Build history of the part. All positions in model axes, mm. A direction names the side the tool comes from. Round coordinates to 2 decimals unless told otherwise and drop trailing zeros. Order: outer loops, then holes, each group sorted by start corner. A loop starts at its lowest first (then second) coordinate and runs counter-clockwise, first axis right, second up. Notation, with made-up numbers: (1, 62.5) -> (59, 62.5) arc R10 ccw to (59, 66.5) -> close; hole circle Ø2 at (1, 7). An arc over 180 degrees is marked (long way). Use a Markdown table: item, result. Add a question column.
Item 1: Pin check, flat tips, straight feed: pin 1 (5 mm diameter, centred on x = -35.5, y = -16.5, fed in from -Z); pin 2 (4.5 mm diameter, centred on y = -19.5, z = 21.5, fed in from +X); pin 3 (14 mm diameter, centred on y = -8.5, z = 2, fed in from +X); pin 4 (12 mm diameter, centred on x = -6.5, z = 8.5, fed in from -Y). Stop position of each tip, or through.
Item 2: Slice it at C-C, the plane z = -11.5. Give the cut face in (x, y).
Item 3: Slice it at D-D, the plane y = -21.5. Give the cut face in (x, z), plus the area to 3 significant figures.
Item 4: 3-axis set-ups, long thin cutter, end or side, ignore diameter. For faces 4 (the face through (59.6, -12.52, -59.68)), 5 (the face through (-18.904, -6, 0)), 6 (the face through (21, -12.7, 0)), 7 (the face through (42.93, -12.52, 37.37)), 8 (the face through (-43.47, -12.52, 37.91)): which of +Z, -Z, +X, -X, +Y, -Y reach the whole face in a straight line?
Item 5: Slice it at B-B, the plane x = 2.5. Give the cut face in (y, z), plus the area to 3 significant figures.
Item 6: Two-plate mould, pull along Z, no slides. Class faces 1 (the face through (-37.37, -12.52, 42.93)), 2 (the face through (0, 0, 23)), 3 (the face through (0, -6, -18.904)): released by +Z, released by -Z, zero draft, split by the parting line, or undercut.
Item 7: Probe L1, parallel to X at y = -11, z = -8; L2, parallel to X at y = -23, z = 33. List the from-to ranges inside material, lowest first.
Item 8: Slice it at A-A, the plane y = -10.5. Give the cut face in (x, z).
from build123d import *

# Parameters (mm, degrees)
F0_W     = 37.8080839926
F0_H     = 37.8080839926
F1_DEPTH = 12.7
F4_DEPTH = 25.4


# Not quite as in the source:
# - the program builds the solid bodies; features that only make, move or delete a surface that nothing else refers to are left out


with BuildPart() as f1:
    # F0 (on Front) → F1 (new body)
    with BuildSketch(Plane.XZ):
        Polygon((23.9840419963, 18.4223433702), (23.9840419963, 23.9840419963), (18.4223433702, 23.9840419963), (-18.4223433702, 23.9840419963), (-23.9840419963, 23.9840419963), (-23.9840419963, 18.4223433702), (-23.9840419963, -18.4223433702), (-23.9840419963, -23.9840419963), (-18.4223433702, -23.9840419963), (18.4223433702, -23.9840419963), (23.9840419963, -23.9840419963), (23.9840419963, -18.4223433702), align=None)
        Rectangle(F0_W, F0_H, mode=Mode.SUBTRACT)
    extrude(amount=F1_DEPTH)

    # F0 (on Front) → F4 (join)
    with BuildSketch(Plane.XZ):
        with BuildLine():
            Line((-23.9840419963, 23.9840419963), (-18.4223433702, 23.9840419963))
            Line((-18.4223433702, 23.9840419963), (-44.0913446559, 49.653043282))
            ThreePointArc((-44.0913446559, 49.653043282), (-46.5728804881, 46.5728804881), (-49.653043282, 44.0913446559))
            Line((-49.653043282, 44.0913446559), (-23.9840419963, 18.4223433702))
            Line((-23.9840419963, 18.4223433702), (-23.9840419963, 23.9840419963))
        make_face()
        with BuildLine():
            ThreePointArc((-49.653043282, 44.0913446559), (-46.5728804881, 46.5728804881), (-44.0913446559, 49.653043282))
            Line((-44.0913446559, 49.653043282), (-56.85978783, 62.4214864561))
            Line((-56.85978783, 62.4214864561), (-62.4214864561, 56.85978783))
            Line((-62.4214864561, 56.85978783), (-49.653043282, 44.0913446559))
        make_face()
        with BuildLine():
            ThreePointArc((-44.0913446559, -49.653043282), (-46.5728804881, -46.5728804881), (-49.653043282, -44.0913446559))
            Line((-49.653043282, -44.0913446559), (-62.4214864561, -56.85978783))
            Line((-62.4214864561, -56.85978783), (-56.85978783, -62.4214864561))
            Line((-56.85978783, -62.4214864561), (-44.0913446559, -49.653043282))
        make_face()
        with BuildLine():
            Line((-23.9840419963, -23.9840419963), (-23.9840419963, -18.4223433702))
            Line((-23.9840419963, -18.4223433702), (-49.653043282, -44.0913446559))
            ThreePointArc((-49.653043282, -44.0913446559), (-46.5728804881, -46.5728804881), (-44.0913446559, -49.653043282))
            Line((-44.0913446559, -49.653043282), (-18.4223433702, -23.9840419963))
            Line((-18.4223433702, -23.9840419963), (-23.9840419963, -23.9840419963))
        make_face()
        with BuildLine():
            Line((49.653043282, -44.0913446559), (23.9840419963, -18.4223433702))
            Line((23.9840419963, -18.4223433702), (23.9840419963, -23.9840419963))
            Line((23.9840419963, -23.9840419963), (18.4223433702, -23.9840419963))
            Line((18.4223433702, -23.9840419963), (44.0913446559, -49.653043282))
            ThreePointArc((44.0913446559, -49.653043282), (46.5728804881, -46.5728804881), (49.653043282, -44.0913446559))
        make_face()
        with BuildLine():
            Line((62.4214864561, -56.85978783), (49.653043282, -44.0913446559))
            ThreePointArc((49.653043282, -44.0913446559), (46.5728804881, -46.5728804881), (44.0913446559, -49.653043282))
            Line((44.0913446559, -49.653043282), (56.85978783, -62.4214864561))
            Line((56.85978783, -62.4214864561), (62.4214864561, -56.85978783))
        make_face()
        with BuildLine():
            Line((56.85978783, 62.4214864561), (44.0913446559, 49.653043282))
            ThreePointArc((44.0913446559, 49.653043282), (46.5728804881, 46.5728804881), (49.653043282, 44.0913446559))
            Line((49.653043282, 44.0913446559), (62.4214864561, 56.85978783))
            Line((62.4214864561, 56.85978783), (56.85978783, 62.4214864561))
        make_face()
        with BuildLine():
            Line((18.4223433702, 23.9840419963), (23.9840419963, 23.9840419963))
            Line((23.9840419963, 23.9840419963), (23.9840419963, 18.4223433702))
            Line((23.9840419963, 18.4223433702), (49.653043282, 44.0913446559))
            ThreePointArc((49.653043282, 44.0913446559), (46.5728804881, 46.5728804881), (44.0913446559, 49.653043282))
            Line((44.0913446559, 49.653043282), (18.4223433702, 23.9840419963))
        make_face()
    extrude(amount=F4_DEPTH)


solid = f1.part
Check sheet entries:
| question | item | result |
|---|---|---|
| 1 | pin 1 | z = -43.56 |
| 1 | pin 2 | x = 29.31 |
| 1 | pin 3 | x = 23.98 |
| 1 | pin 4 | through |
| 2 | outline | (-23.98, -12.7) -> (-18.9, -12.7) -> (-18.9, 0) -> (-23.98, 0) -> close; (18.9, -12.7) -> (23.98, -12.7) -> (23.98, 0) -> (18.9, 0) -> close |
| 3 | outline | (-62.42, -56.86) -> (-56.86, -62.42) -> (-18.42, -23.98) -> (-23.98, -23.98) -> (-23.98, -18.42) -> close; (-62.42, 56.86) -> (-23.98, 18.42) -> (-23.98, 23.98) -> (-18.42, 23.98) -> (-56.86, 62.42) -> close; (18.42, -23.98) -> (56.86, -62.42) -> (62.42, -56.86) -> (23.98, -18.42) -> (23.98, -23.98) -> close; (18.42, 23.98) -> (23.98, 23.98) -> (23.98, 18.42) -> (62.42, 56.86) -> (56.86, 62.42) -> close |
| 3 | area | 1,650 mm2 |
| 4 | face 4 | -Z, +X, +Y, -Y |
| 4 | face 5 | +Y, -Y |
| 4 | face 6 | -Y |
| 4 | face 7 | +X, +Y, -Y |
| 4 | face 8 | -X, +Y, -Y |
| 5 | outline | (-12.7, -23.98) -> (0, -23.98) -> (0, -18.9) -> (-12.7, -18.9) -> close; (-12.7, 18.9) -> (0, 18.9) -> (0, 23.98) -> (-12.7, 23.98) -> close |
| 5 | area | 129 mm2 |
| 6 | face 1 | released by +Z |
| 6 | face 2 | zero draft |
| 6 | face 3 | undercut |
| 7 | L1 | -23.98 to -18.9, 18.9 to 23.98 |
| 7 | L2 | -38.56 to -27.44, 27.44 to 38.56 |
| 8 | outline | (-62.42, -56.86) -> (-56.86, -62.42) -> (-18.42, -23.98) -> (18.42, -23.98) -> (56.86, -62.42) -> (62.42, -56.86) -> (23.98, -18.42) -> (23.98, 18.42) -> (62.42, 56.86) -> (56.86, 62.42) -> (18.42, 23.98) -> (-18.42, 23.98) -> (-56.86, 62.42) -> (-62.42, 56.86) -> (-23.98, 18.42) -> (-23.98, -18.42) -> close; hole (-18.9, -18.9) -> (18.9, -18.9) -> (18.9, 18.9) -> (-18.9, 18.9) -> close |
